Geometry: final body of the model. Coordinates: model frame, mm. Face numbers are marked on the shaded views. A direction names the side the tool comes from. Coordinates: 2 decimals unless noted, no trailing zeros. Write each loop counter-clockwise with the first axis right and the second up, starting at its lowest first coordinate (ties: lowest second). Pieces come first, ordered by that corner, then holes. Notation, with made-up numbers: (-21, 4.5) - (14, 4.5) arc R20 cw to (14, 10.5) - close; hole circle Ø7 at (53, 8.25). An arc over 180 degrees is marked (long way). Put each result on its own line as item: value.
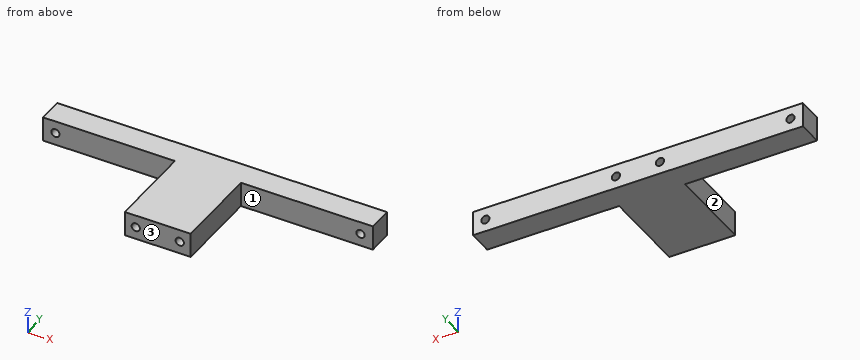
```python
from build123d import *

# Parameters (mm, degrees)
SKETCH1_W           = 381
SKETCH1_H           = 28.575
SKETCH1_W_2         = 76.2
SKETCH1_H_2         = 101.6
BOSS_EXTRUDE1_DEPTH = 28.575
SKETCH2_R           = 4.7625
CUT_EXTRUDE1_DEPTH  = 233.491529416


with BuildPart() as part:
    # Sketch1 → Boss-Extrude1 (new body)
    with BuildSketch(Plane.XY):
        with Locations((0, -14.2875)):
            Rectangle(SKETCH1_W, SKETCH1_H)
        with Locations((0, -79.375)):
            Rectangle(SKETCH1_W_2, SKETCH1_H_2)
    extrude(amount=BOSS_EXTRUDE1_DEPTH)

    # Sketch2 → Cut-Extrude1 (cut, through all)
    with BuildSketch(Plane(origin=(0, 0, 0), x_dir=(1, 0, 0), z_dir=(0, 1, 0))):
        with Locations(Location((-176.2125, -14.2875, 0), (0, 0, 270))):
            Circle(SKETCH2_R)
        with Locations(Location((-25.4, -14.2875, 0), (0, 0, 270))):
            Circle(SKETCH2_R)
        with Locations(Location((25.4, -14.2875, 0), (0, 0, 90))):
            Circle(SKETCH2_R)
        with Locations(Location((176.2125, -14.2875, 0), (0, 0, 270))):
            Circle(SKETCH2_R)
    extrude(amount=-CUT_EXTRUDE1_DEPTH, mode=Mode.SUBTRACT)


solid = part.part
```
1. Section query B-B (y = -18). Count the separate pieces of the cut face and the enclosed holes in it, then the cut area to 3 significant figures.
Answer below:
separate pieces: 1
enclosed holes: 4
area: 10,600 mm²
2. Section query A-A (x = 25.4). Return loops of the section in (y, z) (3 decimals), then the cut area to 3 significant figures.
Answer below:
outline: (-130.175, 0) - (0, 0) - (0, 9.525) - (-130.175, 9.525) - close; (-130.175, 19.05) - (0, 19.05) - (0, 28.575) - (-130.175, 28.575) - close
area: 2,480 mm²
3. Section query C-C (z = 24.25). Return loops of the section in (x, y) (3 decimals), then the cut area to 3 significant figures.
Answer below:
outline: (-190.5, -28.575) - (-38.1, -28.575) - (-38.1, -130.175) - (38.1, -130.175) - (38.1, -28.575) - (190.5, -28.575) - (190.5, 0) - (-190.5, 0) - close
area: 18,600 mm²
4. Pin query (flat end, axial travel): pin 1 Ø14.5 at (x, z) = (-101.5, 9) entering from -Y (3 decimals); pin 2 Ø8 at (y, z) = (-57.5, 23) entering from +X; pin 3 Ø14.5 at (y, z) = (-73.5, 12.5) entering from -X. Return the tip coordinate at first contact, or that it passes through.
Answer below:
pin 1: stops at y = -28.575
pin 2: stops at x = 38.1
pin 3: stops at x = -38.1
5. Set-up query: the marked faces 1, 2 and 3. Return all of +Z, -Z, +X, -X, +Y, -Y with unobstructed straight access to the full face (end or side cutting, diameter ignored); none if empty.
Answer below:
face 1: +Z, -Z, +X, -Y
face 2: +Z, -Z, -X, -Y
face 3: +Z, -Z, +X, -X, -Y
6. Ray query, probe 1 along X at (y, z) = (-42.5, 15.25); probe 2 along X at (y, z) = (-81.5, 11.5); probe 3 along Z at (x, y) = (25.4, -62.5) (3 decimals). Return the intervals inside material, ascending. Write a range as from..to.
Answer below:
probe 1: x = -38.1..-30.06, -20.74..20.74, 30.06..38.1
probe 2: x = -38.1..-29.26, -21.54..21.54, 29.26..38.1
probe 3: z = 0..9.525, 19.05..28.575
